Check sheet for the modelled part. Datum: model origin and axes. Units: mm. A direction names the side the tool comes from. Give positions to 0.01 mm unless a question says otherwise; leave off trailing zeros. Order: outer loops, then holes, each group sorted by start corner. A loop starts at its lowest first (then second) coordinate and runs counter-clockwise, first axis right, second up.
Item 1: Sectioned sample at D-D on y = -7. Record the boundary of the cut face in (x, z), and give its area (3 significant figures).
Item 2: Release check for a two-part mould opening along X. For faces 3 (the cylindrical face through (9.76, -2.17, 7.6)), 4 (the flat face through (-15.97, 51.29, 7.4)), 5 (the flat face through (0, -11, 15)) record: released by +X, released by -X, zero draft, split by the parting line, or undercut.
Item 3: Sectioned sample at A-A on x = 0. Record the boundary of the cut face in (y, z), and give its area (3 significant figures).
Item 4: Material ranges on line 1 along Y through (x, z) = (-0.5, 6); line 2 along X through (y, z) = (75, 7.25); line 3 along Y through (x, z) = (-5.5, 11.25), recorded low to high.
Item 5: Gauge pin test, flat ends, axial feed: P1, Ø2, axis at x = -21, z = 7, coming from the -Y side; P2, Ø6, axis at y = 12, z = 6.5, coming from the -X side. Record the tip position at first contact, or that the pin passes through.
Item 6: Sectioned sample at B-B on y = 77.5. Record the boundary of the cut face in (x, z).
Item 7: Access from +Z, -Z, +X, -X, +Y, -Y to the whole of each face (thin tool, end or side, straight path). Record for faces 1 (the flat face through (52.4, -11.81, 7.4)), 2 (the flat face through (-36.429, -39.475, 7.395)).
Item 8: Sectioned sample at C-C on z = 7.5. Record the boundary of the cut face in (x, y).
Autodesk Fusion 360 part; units mm, degrees
sketch "Skizze1" plane through (0, 0, 0) normal (0, 0, 1) x (1, 0, 0)
  circle A0 centre (0, 0) radius 25
  circle A1 centre (0, 75) radius 12.5
  line L0 (0, 0) -> (21.6506, 12.5) construction
  line L1 (0, 0) -> (25, 0) construction
  line L2 (21.6506, 12.5) -> (12.5, 75)
  line L3 (0, 0) -> (-21.6506, 12.5) construction
  line L4 (-21.6506, 12.5) -> (-12.5, 75)
  line L5 (0, 75) -> (0, 0) construction
  line L6 (0, 75) -> (-12.5, 75) construction
  line L7 (0, 75) -> (12.5, 75) construction
  line L8 (-21.6506, 12.5) -> (-71.2019, -26.6747)
  circle A2 centre (-64.9519, -37.5) radius 12.5
  line L9 (0, -25) -> (-58.7019, -48.3253)
  line L10 (0, -25) -> (58.7019, -48.3253)
  circle A3 centre (64.9519, -37.5) radius 12.5
  line L11 (21.6506, 12.5) -> (71.2019, -26.6747)
  dimension "d1" = 50
  dimension "d3" = 25
  dimension "d4" = 30
  dimension "d5" = 30
  dimension "d6" = 75
  dimension "d10" = 360
extrude "Extrusion1" add sketch "Skizze1" along normal blind 15
fillet "Abrundung1" radius 40 3 edges at (-21.6506, 12.5, 7.5) (0, -25, 7.5) (21.6506, 12.5, 7.5)
sketch "Skizze2" plane through (0, 0, 0) normal (0, 0, -1) x (-1, 0, 0)
  arc A0 (12.5, 75) -> (-12.5, 75) centre (0, 75) ccw
  line L0 (-12.5, 75) -> (-19.3481, 28.2264)
  arc A1 (-34.1189, 2.6428) -> (-19.3481, 28.2264) centre (-58.9262, 34.021) ccw
  line L1 (-34.1189, 2.6428) -> (-71.2019, -26.6747)
  arc A2 (-71.2019, -26.6747) -> (-58.7019, -48.3253) centre (-64.9519, -37.5) ccw
  line L2 (-58.7019, -48.3253) -> (-14.7707, -30.8692)
  arc A3 (14.7707, -30.8692) -> (-14.7707, -30.8692) centre (0, -68.0421) ccw
  line L3 (14.7707, -30.8692) -> (58.7019, -48.3253)
  arc A4 (58.7019, -48.3253) -> (71.2019, -26.6747) centre (64.9519, -37.5) ccw
  line L4 (71.2019, -26.6747) -> (34.1189, 2.6428)
  arc A5 (19.3481, 28.2264) -> (34.1189, 2.6428) centre (58.9262, 34.021) ccw
  line L5 (19.3481, 28.2264) -> (12.5, 75)
  point P0 (0, 75)
  point P1 (-64.9519, -37.5)
  point P2 (64.9519, -37.5)
hole "Bohrung1" at (0, 75, 0) at (-64.9519, -37.5, 0) at (64.9519, -37.5, 0) direction (0, 0, 1) diameter 10 end through all
sketch "Skizze4" plane through (0, 0, 0) normal (0, 0, -1) x (-1, 0, 0)
  circle A0 centre (64.9519, -37.5) radius 5
  circle A1 centre (0, 75) radius 5
  circle A2 centre (-64.9519, -37.5) radius 5
  arc A3 (12.5, 75) -> (-12.5, 75) centre (0, 75) ccw
  line L0 (-12.5, 75) -> (-19.3481, 28.2264)
  arc A4 (-34.1189, 2.6428) -> (-19.3481, 28.2264) centre (-58.9262, 34.021) ccw
  line L1 (-34.1189, 2.6428) -> (-71.2019, -26.6747)
  arc A5 (-71.2019, -26.6747) -> (-58.7019, -48.3253) centre (-64.9519, -37.5) ccw
  line L2 (-58.7019, -48.3253) -> (-14.7707, -30.8692)
  arc A6 (14.7707, -30.8692) -> (-14.7707, -30.8692) centre (0, -68.0421) ccw
  line L3 (14.7707, -30.8692) -> (58.7019, -48.3253)
  arc A7 (58.7019, -48.3253) -> (71.2019, -26.6747) centre (64.9519, -37.5) ccw
  line L4 (71.2019, -26.6747) -> (34.1189, 2.6428)
  arc A8 (19.3481, 28.2264) -> (34.1189, 2.6428) centre (58.9262, 34.021) ccw
  line L5 (19.3481, 28.2264) -> (12.5, 75)
hole "Bohrung2" at (0, 0, 0) direction (0, 0, 1) diameter 20 end through all
Report:
1. outline: (-46.32, 0) - (-7.14, 0) - (-7.14, 15) - (-46.32, 15) - close; (7.14, 0) - (46.32, 0) - (46.32, 15) - (7.14, 15) - close
1. area: 1,180 mm2
2. face 3: undercut
2. face 4: released by -X
2. face 5: zero draft
3. outline: (-28.04, 0) - (-10, 0) - (-10, 15) - (-28.04, 15) - close; (10, 0) - (70, 0) - (70, 15) - (10, 15) - close; (80, 0) - (87.5, 0) - (87.5, 15) - (80, 15) - close
3. area: 1,280 mm2
4. line 1: y = -28.05 to -9.99, 9.99 to 70.03, 79.97 to 87.49
4. line 2: x = -12.5 to -5, 5 to 12.5
4. line 3: y = -28.42 to -8.35, 8.35 to 86.22
5. P1: stops at y = -33.74
5. P2: stops at x = -27.72
6. outline: (-12.25, 0) - (-4.33, 0) - (-4.33, 15) - (-12.25, 15) - close; (4.33, 0) - (12.25, 0) - (12.25, 15) - (4.33, 15) - close
7. face 1: +Z, -Z, +X, +Y
7. face 2: +Z, -Z, -Y
8. outline: (-71.2, -26.67) arc R12.5 ccw to (-58.7, -48.33) - (-14.77, -30.87) arc R40 cw to (14.77, -30.87) - (58.7, -48.33) arc R12.5 ccw to (71.2, -26.67) - (34.12, 2.64) arc R40 cw to (19.35, 28.23) - (12.5, 75) arc R12.5 ccw to (-12.5, 75) - (-19.35, 28.23) arc R40 cw to (-34.12, 2.64) - close; hole circle Ø10 at (-64.95, -37.5); hole circle Ø20 at (0, 0); hole circle Ø10 at (0, 75); hole circle Ø10 at (64.95, -37.5)
